```python
from build123d import *

# Parameters (mm, degrees)
F1_W     = 16
F1_H     = 22
F1_W_2   = 10
F1_H_2   = 20
F2_DEPTH = 2
F3_SIZE2 = 1
F3_SIZE  = 1
F4_SIZE2 = 1
F4_SIZE  = 1
F5_R     = 0.2


with BuildPart() as f2:
    # F1 (on face) → F2 (new body)
    with BuildSketch(Plane.XY):
        Rectangle(F1_W, F1_H)
        Rectangle(F1_W_2, F1_H_2, mode=Mode.SUBTRACT)
    extrude(amount=F2_DEPTH)

    # F3
    f3_edges = [f2.edges().sort_by_distance(p)[0] for p in [
        (-8, -11, 1),
    ]]
    chamfer(f3_edges, length=F3_SIZE, length2=F3_SIZE2)

    # F4
    f4_edges = [f2.edges().sort_by_distance(p)[0] for p in [
        (8, -11, 1),
        (8, 11, 1),
        (-8, 11, 1),
    ]]
    chamfer(f4_edges, length=F4_SIZE, length2=F4_SIZE2)

    # F5
    f5_edges = [f2.edges().sort_by_distance(p)[0] for p in [
        (-8, 0, 2),
        (-7.5, 10.5, 2),
        (-7.5, -10.5, 2),
        (0, 11, 2),
        (0, -11, 2),
        (7.5, 10.5, 2),
        (7.5, -10.5, 2),
        (8, 0, 2),
        (-5, 0, 2),
        (0, 10, 2),
        (5, 0, 2),
        (0, -10, 2),
        (-8, 0, 0),
        (-7.5, 10.5, 0),
        (-7.5, -10.5, 0),
        (0, 11, 0),
        (0, -11, 0),
        (7.5, 10.5, 0),
        (7.5, -10.5, 0),
        (8, 0, 0),
        (-5, 0, 0),
        (0, 10, 0),
        (5, 0, 0),
        (0, -10, 0),
    ]]
    fillet(f5_edges, radius=F5_R)


solid = f2.part
```
Verification items for the finished model (mm, model axes). A direction names the side the tool comes from. Give positions to 0.01 mm unless a question says otherwise; leave off trailing zeros. Loops run counter-clockwise (first coordinate to the right, second up) from the corner with the lowest first, then second, coordinate; pieces in that order, holes last. Notation, with made-up numbers: M -33.5,60 L -15.5,60 A20 cw -15.5,77 Z; hole C -27.5,-15 d6. An arc over 180 degrees is marked long. Return JSON: item names as keys, results as strings.
1) Mould release check, pull along X, two halves, no side actions. Record for faces 1 (the flat face through (0, -10, 1)), 2 (the flat face through (7.5, 10.5, 1)), 3 (the flat face through (-7.5, -10.5, 1)): released by +X, released by -X, zero draft, split by the parting line, or undercut.
Findings:
{"face 1": "undercut", "face 2": "released by +X", "face 3": "released by -X"}
2) Tool access check on faces 4 (the flat face through (8, 0, 1)), 5 (the flat face through (5, 0, 1)). Record the directions out of +Z, -Z, +X, -X, +Y, -Y that give a thin tool (end or side, any length) a straight path to the whole face; none if there is none.
Findings:
{"face 4": "+Z, -Z, +X, +Y, -Y", "face 5": "+Z, -Z"}
3) Section check A-A, the plane x = -3. Enter the section's corners in (y, z).
Findings:
{"outline": "M -11,0.2 A0.2 ccw -10.8,0 L -10.2,0 A0.2 ccw -10,0.2 L -10,1.8 A0.2 ccw -10.2,2 L -10.8,2 A0.2 ccw -11,1.8 Z; M 10,0.2 A0.2 ccw 10.2,0 L 10.8,0 A0.2 ccw 11,0.2 L 11,1.8 A0.2 ccw 10.8,2 L 10.2,2 A0.2 ccw 10,1.8 Z"}
4) Section check C-C, the plane z = 1.45. Enter the section's corners in (x, y), and give its area (3 significant figures).
Findings:
{"outline": "M -8,-10 L -7,-11 L 7,-11 L 8,-10 L 8,10 L 7,11 L -7,11 L -8,10 Z; hole M -5,-10 L 5,-10 L 5,10 L -5,10 Z", "area": "150 mm2"}
5) Section check B-B, the plane y = -3.25. Enter the section's corners in (x, z), and give its area (3 significant figures).
Findings:
{"outline": "M -8,0.2 A0.2 ccw -7.8,0 L -5.2,0 A0.2 ccw -5,0.2 L -5,1.8 A0.2 ccw -5.2,2 L -7.8,2 A0.2 ccw -8,1.8 Z; M 5,0.2 A0.2 ccw 5.2,0 L 7.8,0 A0.2 ccw 8,0.2 L 8,1.8 A0.2 ccw 7.8,2 L 5.2,2 A0.2 ccw 5,1.8 Z", "area": "11.9 mm2"}
6) Gauge pin test, flat end, axial feed: P1, Ø3, axis at x = 0.5, y = -7, coming from the -Z side. Record the tip position at first contact, or that the pin passes through.
Findings:
{"P1": "passes through"}
7) Material ranges on L1, parallel to X at y = 9.5, z = 1; L2, parallel to Y at x = -3, z = 0.7; L3, parallel to Y at x = 6, z = 1.85, recorded low to high. Write a range as [from, to].
Findings:
{"L1": "x = [-8, -5], [5, 8]", "L2": "y = [-11, -10], [10, 11]", "L3": "y = [-10.99, 10.99]"}
